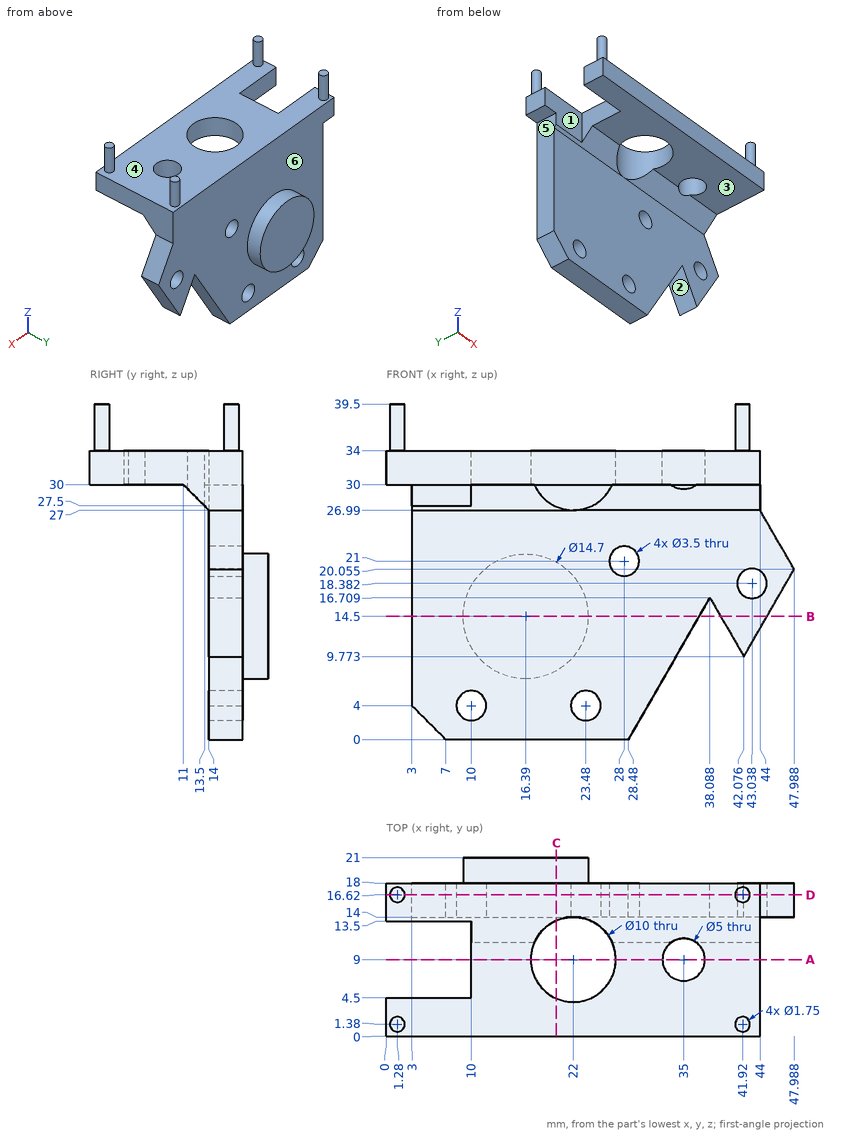
Answer from the drawing. Dimensions are ordinates in mm from the lowest x, y and z of the part. A direction names the side the tool comes from. Round coordinates to 2 decimals unless told otherwise and drop trailing zeros. Write each loop counter-clockwise with the first axis right and the second up, starting at its lowest first coordinate (ties: lowest second). Pieces come first, ordered by that corner, then holes. Notation, with made-up numbers: M 39,-35 L 76,-35 A18 cw 76,-10 Z; hole C 9.5,-3 d9. An arc over 180 degrees is marked long. Write each question's results on one line, items separated by ' | '. Start each with the question number.
Item 1: A cutting plane is placed at C-C on x = 20. Write down the section's boundary in (y, z).
Item 2: For the marked faces 1, 2 and 3, determine the directions among +Z, -Z, +X, -X, +Y, -Y from which every point of the face is accessible in a straight line to the end or side of a thin tool.
Item 3: Flat-ended cylindrical pins translate along their axes: pin 1 Ø1 at (x, y) = (31.5, 15.5) entering from -Z (1 decimal); pin 2 Ø2 at (y, z) = (11, 30.5) entering from +X; pin 3 Ø1.5 at (y, z) = (15.5, 35) entering from +X; pin 4 Ø12 at (x, y) = (19, 11.5) entering from -Z. Find the tip coordinate at first contact, or state that the pin passes through.
Item 4: A cutting plane is placed at A-A on y = 9. Write down the section's boundary in (x, z).
Item 5: A cutting plane is placed at D-D on y = 16.62. State how many separate pieces and enclosed holes the cut face has, and give its area (3 significant figures).
Item 6: A cutting plane is placed at B-B on z = 14.5. Write down the section's boundary in (x, y).
Item 7: For a pull along X with two mould halves and no side action, classify the marked faces 4, 5 and 6 as pulls with the +X half, pulls with the -X half, needs draft (parallel to the pull), parting line crosses it, or undercut.
Item 8: Straight lines are drawn through the part: L1, parallel to X at y = 9, z = 31.15; L2, parallel to Y at x = 35, z = 33.15; L3, parallel to Y at x = 12.5, z = 6. For each, find the intervals that lie inside material, in ascending order. Write a range as [from, to].
Check sheet entries:
1) outline: M 0,30 L 4.42,30 L 4.42,34 L 0,34 Z; M 13.58,27.42 L 14,27 L 14,0 L 18,0 L 18,8.1 L 21,8.1 L 21,20.9 L 18,20.9 L 18,34 L 13.58,34 Z
2) face 1: +Z, -Z, -X | face 2: -Z, +Y, -Y | face 3: -Z, +X, -X, -Y
3) pin 1: z = 4.4 | pin 2: x = 44 | pin 3: x = 42.71 | pin 4: z = 0
4) outline: M 10,30 L 17,30 L 17,34 L 10,34 Z; M 27,30 L 32.5,30 L 32.5,34 L 27,34 Z; M 37.5,30 L 44,30 L 44,34 L 37.5,34 Z
5) separate pieces: 1 | enclosed holes: 4 | area: 1,250 mm²
6) outline: M 3,14 L 36.82,14 L 36.82,18 L 23.74,18 L 23.74,21 L 9.04,21 L 9.04,18 L 3,18 Z; M 39.36,14 L 44.79,14 L 44.79,18 L 39.36,18 Z
7) face 4: undercut | face 5: pulls with the -X half | face 6: needs draft
8) L1: [10, 17], [27, 32.5], [37.5, 44] | L2: [0, 6.5], [11.5, 18] | L3: [14, 18]
